```python
from build123d import *

# Parameters (mm, degrees)
F0_W     = 152.4
F0_H     = 172.72
F0_R     = 1.8288
F1_DEPTH = 3.175
F2_SIZE  = 1.27


with BuildPart() as f1:
    # F0 (on Front) → F1 (new body)
    with BuildSketch(Plane.XZ):
        Rectangle(F0_W, F0_H)
        with BuildLine():
            ThreePointArc((-66.675, -85.0773), (-68.5673, -83.185), (-66.675, -81.2927))
            Line((-66.675, -81.2927), (-47.625, -81.2927))
            ThreePointArc((-47.625, -81.2927), (-45.7327, -83.185), (-47.625, -85.0773))
            Line((-47.625, -85.0773), (-66.675, -85.0773))
        make_face(mode=Mode.SUBTRACT)
        with BuildLine():
            Line((15.875, -85.0773), (-3.175, -85.0773))
            ThreePointArc((-3.175, -85.0773), (-5.0673, -83.185), (-3.175, -81.2927))
            Line((-3.175, -81.2927), (15.875, -81.2927))
            ThreePointArc((15.875, -81.2927), (17.7673, -83.185), (15.875, -85.0773))
        make_face(mode=Mode.SUBTRACT)
        with Locations((38.1, -83.185)):
            Circle(F0_R, mode=Mode.SUBTRACT)
        with Locations((57.15, -83.185)):
            Circle(F0_R, mode=Mode.SUBTRACT)
        with BuildLine():
            Line((-66.675, 85.0773), (-47.625, 85.0773))
            ThreePointArc((-47.625, 85.0773), (-45.7327, 83.185), (-47.625, 81.2927))
            Line((-47.625, 81.2927), (-66.675, 81.2927))
            ThreePointArc((-66.675, 81.2927), (-68.5673, 83.185), (-66.675, 85.0773))
        make_face(mode=Mode.SUBTRACT)
        with BuildLine():
            ThreePointArc((-3.175, 81.2927), (-5.0673, 83.185), (-3.175, 85.0773))
            Line((-3.175, 85.0773), (15.875, 85.0773))
            ThreePointArc((15.875, 85.0773), (17.7673, 83.185), (15.875, 81.2927))
            Line((15.875, 81.2927), (-3.175, 81.2927))
        make_face(mode=Mode.SUBTRACT)
        with Locations((38.1, 83.185)):
            Circle(F0_R, mode=Mode.SUBTRACT)
        with Locations((57.15, 83.185)):
            Circle(F0_R, mode=Mode.SUBTRACT)
    extrude(amount=F1_DEPTH)

    # F2
    f2_edges = [f1.edges().sort_by_distance(p)[0] for p in [
        (55.3212, 0, 83.185),
        (36.2712, 0, 83.185),
        (17.7673, 0, 83.185),
        (6.35, 0, 85.0773),
        (-5.0673, 0, 83.185),
        (6.35, 0, 81.2927),
        (-45.7327, 0, 83.185),
        (-57.15, 0, 85.0773),
        (-57.15, 0, 81.2927),
        (-68.5673, 0, 83.185),
        (-57.15, 0, -81.2927),
        (-45.7327, 0, -83.185),
        (-57.15, 0, -85.0773),
        (-68.5673, 0, -83.185),
        (-5.0673, 0, -83.185),
        (6.35, 0, -81.2927),
        (17.7673, 0, -83.185),
        (6.35, 0, -85.0773),
        (36.2712, 0, -83.185),
        (55.3212, 0, -83.185),
    ]]
    chamfer(f2_edges, length=F2_SIZE)


solid = f1.part
```
Geometry: final body of the model. Coordinates: model frame, mm. Give positions to 0.01 mm unless a question says otherwise; leave off trailing zeros. Order: outer loops, then holes, each group sorted by start corner. A loop starts at its lowest first (then second) coordinate and runs counter-clockwise, first axis right, second up. Notation, with made-up numbers: (83, 41) -> (129, 41) arc R28 ccw to (129, 74) -> close; hole circle Ø3 at (76, 76). An arc over 180 degrees is marked (long way). Write each question's results on one line, items separated by ' | '. Start each with the question number.
1) Section A-A (x = -59.5). Return loops of the section in (y, z) (3 decimals), then the cut area to 3 significant figures.
2) Section B-B (y = -0.5). Count the separate pieces of the cut face and the enclosed holes in it, then the cut area to 3 significant figures.
3) Draft query along X for faces 1 (the flat face through (-1, 0, 1)), 2 (the cylindrical face through (58.894, -2.209, -82.636)). Return one class per face: pulls with the +X half, pulls with the -X half, needs draft (parallel to the pull), parting line crosses it, or undercut.
4) Line query: line 1 (Z direction, x = 57.15, y = -2.7); line 2 (Z direction, x = 8, y = -1.85). Output: solid intervals per line, ascending. Write a range as from..to.
5) First-contact query: pin 1 (2 mm diameter, centred on x = 38.1, z = -83.185, fed in from -Y); pin 2 (6 mm diameter, centred on x = 38.1, z = 83.185, fed in from +Y); pin 3 (5 mm diameter, centred on x = 57.15, z = -83.185, fed in from +Y). Flat tips, straight axial feed; report the tip coordinate or a pass-through.
Calculated:
1) outline: (-3.175, -86.36) -> (0, -86.36) -> (0, -86.347) -> (-1.27, -85.077) -> (-3.175, -85.077) -> close; (-3.175, -81.293) -> (-1.27, -81.293) -> (0, -80.023) -> (0, 80.023) -> (-1.27, 81.293) -> (-3.175, 81.293) -> close; (-3.175, 85.077) -> (-1.27, 85.077) -> (0, 86.347) -> (0, 86.36) -> (-3.175, 86.36) -> close | area: 521 mm2
2) separate pieces: 1 | enclosed holes: 8 | area: 25,700 mm2
3) face 1: needs draft | face 2: undercut
4) line 1: -86.36..-85.01, -81.36..81.36, 85.01..86.36 | line 2: -86.36..-85.08, -81.29..81.29, 85.08..86.36
5) pin 1: through | pin 2: y = -0.1 | pin 3: y = -0.6
